```python
from build123d import *

# Parameters (mm, degrees)
SKETCH1_R           = 1.2500000000000062
SKETCH1_R_2         = 1.2500000000000029
SKETCH1_R_3         = 1.2499999999999978
SKETCH1_R_4         = 1.2499999999999976
BOSS_EXTRUDE1_DEPTH = 5
BOSS_EXTRUDE2_DEPTH = 20
CUT_EXTRUDE1_DEPTH  = 109.36973747315251
FILLET1_R           = 1
FILLET4_R           = 2
FILLET5_R           = 2
FILLET8_R           = 3
FILLET9_R           = 1


with BuildPart() as part:
    # Sketch1 → Boss-Extrude1 (new body)
    with BuildSketch(Plane(origin=(0, 0, 0), x_dir=(1, 0, 0), z_dir=(0, 1, 0))):
        with BuildLine():
            Line((78, -39.99999999999999), (78, -46))
            ThreePointArc((78, -46), (78.5857864376269, -44.58578643762691), (79.99999999999999, -43.99999999999999))
            Line((79.99999999999999, -44), (85.99999999999999, -44))
            ThreePointArc((85.99999999999999, -44), (87.41421356237308, -44.58578643762691), (87.99999999999999, -46))
            Line((87.99999999999999, -46), (88, -9.999999999999998))
            ThreePointArc((88, -9.999999999999998), (85.07106781186548, -2.9289321881345147), (77.99999999999999, -5.33e-15))
            Line((77.99999999999999, 0), (10.000000000000071, 0))
            ThreePointArc((10.000000000000071, 1.78e-15), (2.9289321881345236, -2.9289321881345245), (0, -10.000000000000071))
            Line((1.22e-15, -10.000000000000071), (5.63e-15, -46))
            ThreePointArc((4.88e-15, -46), (0.5857864376269124, -44.58578643762691), (2.000000000000006, -44))
            Line((2.000000000000006, -44), (8.000000000000005, -44))
            ThreePointArc((8.000000000000005, -44), (9.414213562373103, -44.5857864376269), (10.000000000000007, -46))
            Line((10.000000000000007, -46), (10.000000000000007, -39.99999999999999))
            ThreePointArc((10.000000000000007, -39.99999999999999), (11.46446609406727, -36.464466094067255), (15.000000000000007, -34.99999999999999))
            Line((15.000000000000007, -34.99999999999999), (73, -34.99999999999999))
            ThreePointArc((73, -34.99999999999999), (76.53553390593274, -36.464466094067255), (78, -39.99999999999999))
        make_face()
        with Locations(Location((15.000000000000002, -28.999999999999996, 0), (0, 0, 270))):
            Circle(SKETCH1_R, mode=Mode.SUBTRACT)
        with Locations(Location((14.999999999999998, -6, 0), (0, 0, 270))):
            Circle(SKETCH1_R_2, mode=Mode.SUBTRACT)
        with BuildLine():
            ThreePointArc((17.999999999999996, -11.000000000000004), (18.5857864376269, -9.585786437626908), (19.999999999999996, -9))
            Line((19.999999999999996, -9), (68, -9))
            ThreePointArc((68, -9.000000000000005), (69.41421356237309, -9.58578643762691), (70, -11.000000000000004))
            Line((70, -11.000000000000004), (70, -24))
            ThreePointArc((70, -24), (69.41421356237309, -25.414213562373092), (68, -25.999999999999996))
            Line((68, -26.000000000000004), (19.999999999999996, -26))
            ThreePointArc((19.999999999999996, -26), (18.585786437626908, -25.41421356237309), (18.000000000000004, -24))
            Line((18.000000000000004, -24), (17.999999999999996, -11.000000000000004))
        make_face(mode=Mode.SUBTRACT)
        with Locations(Location((73.00000000000001, -28.999999999999993, 0), (0, 0, 270))):
            Circle(SKETCH1_R_3, mode=Mode.SUBTRACT)
        with Locations(Location((73.00000000000001, -6, 0), (0, 0, 270))):
            Circle(SKETCH1_R_4, mode=Mode.SUBTRACT)
    extrude(amount=BOSS_EXTRUDE1_DEPTH)

    # Sketch1_3 → Boss-Extrude2 (add)
    with BuildSketch(Plane(origin=(0, 0, 0), x_dir=(1, 0, 0), z_dir=(0, 1, 0))):
        with BuildLine():
            Line((10.000000000000007, -57.99999999999998), (10.000000000000007, -46))
            ThreePointArc((10.000000000000007, -46), (9.414213562373103, -44.5857864376269), (8.000000000000005, -44))
            Line((8.000000000000005, -44), (2.000000000000006, -44))
            ThreePointArc((2.000000000000006, -44), (0.5857864376269124, -44.58578643762691), (4.88e-15, -46))
            Line((5.63e-15, -46), (7.1e-15, -57.99999999999998))
            ThreePointArc((7.99e-15, -57.99999999999998), (0.5857864376269144, -59.414213562373085), (2.0000000000000218, -60))
            Line((2.0000000000000218, -60), (7.999999999999993, -60))
            ThreePointArc((7.999999999999993, -60), (9.4142135623731, -59.414213562373085), (10.000000000000007, -57.99999999999998))
        make_face()
        with BuildLine():
            ThreePointArc((78, -57.99999999999999), (78.5857864376269, -59.41421356237309), (80, -60))
            Line((80, -60), (86, -60))
            ThreePointArc((86, -60), (87.41421356237309, -59.4142135623731), (87.99999999999999, -57.99999999999999))
            Line((87.99999999999999, -57.99999999999999), (87.99999999999999, -46))
            ThreePointArc((87.99999999999999, -46), (87.41421356237308, -44.58578643762691), (85.99999999999999, -44))
            Line((85.99999999999999, -44), (79.99999999999999, -44))
            ThreePointArc((79.99999999999999, -43.99999999999999), (78.5857864376269, -44.58578643762691), (78, -46))
            Line((78, -46), (78, -57.99999999999999))
        make_face()
    extrude(amount=BOSS_EXTRUDE2_DEPTH)

    # Sketch2 → Cut-Extrude1 (cut, through all)
    with BuildSketch(Plane(origin=(88, 0, 2.544e-14), x_dir=(-2.9e-16, 0, -1), z_dir=(1, 0, -2.9e-16))):
        Polygon((-59.99999999999998, 8.816905616081954), (-60.00000000000003, 20), (-47.93723198019628, 20), (-51.19632430540917, 3.782535807663335), (-56.34341854385401, 4.816905616081951), (-55.53957096656065, 8.816905616081954), align=None)
    extrude(amount=-CUT_EXTRUDE1_DEPTH, mode=Mode.SUBTRACT)

    # Fillet1
    fillet1_edges = [part.edges().sort_by_distance(p)[0] for p in [
        (87.41421356237309, 8.816905616081954, 59.41421356237309),
        (3.55e-15, 8.816905616081954, 56.769785483280344),
        (9.4142135623731, 8.816905616081954, 59.414213562373085),
        (0.585786437626916, 8.816905616081954, 59.414213562373085),
        (10.00000000000001, 8.816905616081954, 56.76978548328034),
        (78.5857864376269, 8.816905616081954, 59.4142135623731),
        (78, 8.816905616081954, 56.76978548328034),
        (88.00000000000001, 8.816905616081954, 56.76978548328034),
        (83, 8.816905616081954, 60.00000000000001),
        (5.000000000000014, 8.816905616081954, 60.00000000000003),
    ]]
    fillet(fillet1_edges, radius=FILLET1_R)

    # Fillet4
    fillet4_edges = [part.edges().sort_by_distance(p)[0] for p in [
        (88, 5, 28),
        (85.07106781186548, 5, 2.928932188134512),
        (44.00000000000003, 5, 0),
        (2.9289321881345245, 5, 2.9289321881345236),
        (3.43e-15, 5, 28.000000000000036),
    ]]
    fillet(fillet4_edges, radius=FILLET4_R)

    # Fillet5
    fillet5_edges = [part.edges().sort_by_distance(p)[0] for p in [
        (10.000000000000007, 5, 43),
        (11.46446609406727, 5, 36.464466094067255),
        (78, 5, 43),
        (76.53553390593274, 5, 36.464466094067255),
        (44, 5, 34.99999999999999),
    ]]
    fillet(fillet5_edges, radius=FILLET5_R)

    # Fillet8
    fillet8_edges = [part.edges().sort_by_distance(p)[0] for p in [
        (83, 20, 47.93723198019631),
        (5.000000000000014, 20, 47.93723198019633),
    ]]
    fillet(fillet8_edges, radius=FILLET8_R)

    # Fillet9
    fillet9_edges = [part.edges().sort_by_distance(p)[0] for p in [
        (5.000000000000014, 3.782535807663335, 51.19632430540922),
        (83, 3.782535807663335, 51.1963243054092),
    ]]
    fillet(fillet9_edges, radius=FILLET9_R)


solid = part.part
```
Could you check a few things on this model? Use its own coordinates, in mm. A direction names the side the tool comes from. Give positions to 0.01 mm unless a question says otherwise; leave off trailing zeros. Write each loop counter-clockwise with the first axis right and the second up, starting at its lowest first coordinate (ties: lowest second). Pieces come first, ordered by that corner, then holes. Notation, with made-up numbers: (-1, 18) - (25, 18) arc R26 cw to (25, 33) - close; hole circle Ø10 at (43.25, -10.75). An arc over 180 degrees is marked (long way). One line per item, written item: value. Start each with the question number.
Item 1: If we mould it in two halves opening along Z, with no side actions, what happens to faces 6 (the face through (5.07, 11.27, 49.69)), 7 (the face through (87.4, 4.43, 27.75)), 8 (the face through (43.52, 4.43, 0.6))? For each: +Z half, -Z half, draft (parallel to the pull), parting line (faces both ways), or undercut.
Item 2: Imagine slicing it at A-A, the plane z = 29. List the corners of the cut face in (x, y) for me.
Item 3: Imagine slicing it at B-B, the plane x = 63. List the corners of the cut face in (y, z) for me.
Item 4: Imagine slicing it at D-D, the plane z = 6. Give the number of separate pieces and of enclosed holes in the cut face, and give its area (3 significant figures).
Item 5: Please list where these lines run through material, in increasing order: line 1 (X direction, y = 4, z = 29.5); line 2 (Y direction, x = 13, z = 7.5); line 3 (X direction, y = 3.2, z = 6). Write a range as from..to.
Item 6: I'm going to push flat-ended pins straight in: pin 1 (3 mm diameter, centred on x = 84, z = 56.5, fed in from +Y); pin 2 (4 mm diameter, centred on x = 15, z = 6, fed in from -Y); pin 3 (5 mm diameter, centred on x = 6, y = 13.5, fed in from -Z); pin 4 (1.5 mm diameter, centred on y = 9.5, z = 43.5, fed in from -X). Where does each tip first touch, or does it pass through?
Item 7: Imagine slicing it at C-C, the plane y = 15.5. List the corners of the cut face in (x, z) for me.
Item 8: Which directions (+Z, -Z, +X, -X, +Y, -Y) give clear straight access to the entire face, cutting with the end or side of a thin tool? Please do faces 1 (the face through (0.6, 4.43, 28.25)), 2 (the face through (5.07, 4.392, 54.231)), 3 (the face through (83, 8.817, 57)), 4 (the face through (83, 12, 44)), 5 (the face through (78.57, 3.85, 59.4)).
Geometry says:
1. face 6: undercut
1. face 7: draft
1. face 8: -Z half
2. outline: (0, 0) - (13.75, 0) - (13.75, 5) - (2, 5) arc R2 ccw to (0, 3) - close; (16.25, 0) - (71.75, 0) - (71.75, 5) - (16.25, 5) - close; (74.25, 0) - (88, 0) - (88, 3) arc R2 ccw to (86, 5) - (74.25, 5) - close
3. outline: (0, 0) - (3, 0) arc R2 ccw to (5, 2) - (5, 9) - (0, 9) - close; (0, 26) - (5, 26) - (5, 33) arc R2 ccw to (3, 35) - (0, 35) - close
4. separate pieces: 3
4. enclosed holes: 0
4. area: 405 mm^2
5. line 1: 0.27..13.85, 16.15..71.85, 74.15..87.73
5. line 2: 0..5
5. line 3: 0.85..13.75, 16.25..71.75, 74.25..87.15
6. pin 1: y = 8.82
6. pin 2: y = 0
6. pin 3: z = 44
6. pin 4: x = 1.03
7. outline: (0, 46) arc R2 ccw to (2, 44) - (8, 44) arc R2 ccw to (10, 46) - (10, 48.84) - (0, 48.84) - close; (78, 46) arc R2 ccw to (80, 44) - (86, 44) arc R2 ccw to (88, 46) - (88, 48.84) - (78, 48.84) - close
8. face 1: -Z, -X, +Y
8. face 2: +X, -X
8. face 3: +Z, +X, -X, +Y
8. face 4: -Z, +X, -X, +Y
8. face 5: +Z, +Y, -Y
